from build123d import *

# Parameters (mm, degrees)
SKETCH1_W           = 279.4
SKETCH1_H           = 177.8
BOSS_EXTRUDE1_DEPTH = 25.654
SKETCH9_R           = 3.96875
CUT_EXTRUDE1_DEPTH  = 38.1
SKETCH9_7_R         = 2.5
SKETCH9_7_R_2       = 3.96875
BOSS_EXTRUDE2_DEPTH = 49.53
SKETCH13_W          = 127.6
SKETCH13_H          = 108.000000046
BOSS_EXTRUDE3_DEPTH = 49.53
SKETCH14_W          = 73
SKETCH14_H          = 49.53
BOSS_EXTRUDE4_DEPTH = 30.48
FILLET1_R           = 25.4
FILLET2_R           = 25.4


with BuildPart() as part:
    # Sketch1 → Boss-Extrude1 (new body)
    with BuildSketch(Plane(origin=(0, 0, 0), x_dir=(1, 0, 0), z_dir=(0, 1, 0))):
        with Locations((139.7, 88.9)):
            Rectangle(SKETCH1_W, SKETCH1_H)
    extrude(amount=BOSS_EXTRUDE1_DEPTH)

    # Sketch9 → Cut-Extrude1 (cut)
    with BuildSketch(Plane(origin=(0, 25.654, 0), x_dir=(1, 0, 0), z_dir=(0, 1, 0))):
        with Locations((215, 143)):
            Circle(SKETCH9_R)
    extrude(amount=-CUT_EXTRUDE1_DEPTH, mode=Mode.SUBTRACT)

    # Sketch9<7> → Boss-Extrude2 (add)
    with BuildSketch(Plane(origin=(0, 25.654, 0), x_dir=(1, 0, 0), z_dir=(0, 1, 0))):
        Polygon((0, 108.000000046), (127.6, 108.000000046), (127.6, 0), (280, 0), (280, 178), (0, 178), align=None)
        with Locations((35.318924397, 143)):
            Circle(SKETCH9_7_R, mode=Mode.SUBTRACT)
        with Locations((14, 143)):
            Circle(SKETCH9_7_R_2, mode=Mode.SUBTRACT)
        with Locations((68, 143)):
            Circle(SKETCH9_7_R_2, mode=Mode.SUBTRACT)
        with Locations((270, 167)):
            Circle(SKETCH9_7_R_2, mode=Mode.SUBTRACT)
        with Locations((215, 143)):
            Circle(SKETCH9_7_R_2, mode=Mode.SUBTRACT)
        with BuildLine():
            Line((129.639279667, 129.22), (129.639279667, 126.383968902))
            ThreePointArc((129.639279667, 126.383968902), (148.28, 150), (129.639279667, 173.616031098))
            Line((129.639279667, 173.616031098), (129.639279667, 170.78))
            Line((129.639279667, 170.78), (118.360720333, 170.78))
            Line((118.360720333, 170.78), (118.360720333, 173.616031098))
            ThreePointArc((118.360720333, 173.616031098), (99.72, 150), (118.360720333, 126.383968902))
            Line((118.360720333, 126.383968902), (118.360720333, 129.22))
            Line((118.360720333, 129.22), (129.639279667, 129.22))
        make_face(mode=Mode.SUBTRACT)
    extrude(amount=BOSS_EXTRUDE2_DEPTH)

    # Sketch13 → Boss-Extrude3 (add)
    with BuildSketch(Plane(origin=(0, 25.654, 0), x_dir=(1, 0, 0), z_dir=(0, 1, 0))):
        with Locations((63.8, 54.000000023)):
            Rectangle(SKETCH13_W, SKETCH13_H)
    extrude(amount=BOSS_EXTRUDE3_DEPTH)

    # Sketch14 → Boss-Extrude4 (add)
    with BuildSketch(Plane(origin=(0, 0, -178), x_dir=(-1, 0, 0), z_dir=(0, 0, -1))):
        with Locations((-148.500000008, 50.419)):
            Rectangle(SKETCH14_W, SKETCH14_H)
    extrude(amount=BOSS_EXTRUDE4_DEPTH)

    # Fillet1
    fillet1_edges = [part.edges().sort_by_distance(p)[0] for p in [
        (185.000000008, 50.419, -208.48),
    ]]
    fillet(fillet1_edges, radius=FILLET1_R)

    # Fillet2
    fillet2_edges = [part.edges().sort_by_distance(p)[0] for p in [
        (112.000000008, 50.419, -208.48),
    ]]
    fillet(fillet2_edges, radius=FILLET2_R)


solid = part.part
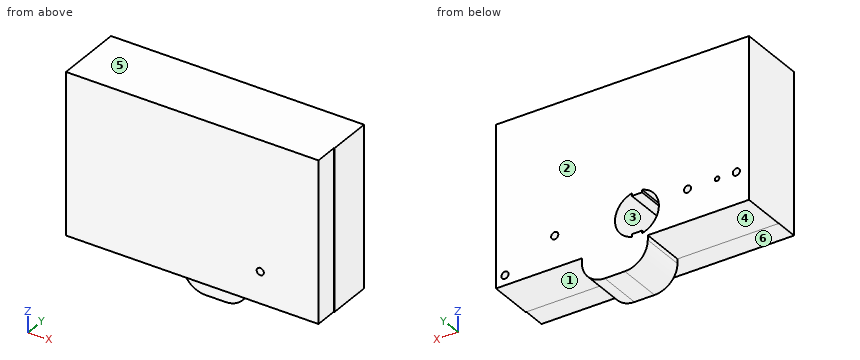
The listing builds one solid part. Answer for the finished solid, in the listing's coordinates (mm). Face numbers are marked on the shaded views. A direction names the side the tool comes from. Coordinates: 2 decimals unless noted, no trailing zeros. Write each loop counter-clockwise with the first axis right and the second up, starting at its lowest first coordinate (ties: lowest second). Pieces come first, ordered by that corner, then holes. Notation, with made-up numbers: M 87,-8 L 117,-8 A23 ccw 117,2 Z; hole C -29,52.25 d9. An arc over 180 degrees is marked long. Put each result on its own line as item: value. Start each with the question number.
1. A cutting plane is placed at B-B on y = 70. Write down the section's boundary in (x, z), then the cut area to 3 significant figures.
2. Consider line 1 (X direction, y = 20, z = -143); line 2 (X direction, y = 46, z = -143); line 3 (Z direction, x = 68, y = 50). Determine where each line is inside the solid, lowest interval first. Write a range as from..to.
3. For a pull along Z with two mould halves and no side action, classify the marked faces 1, 2 and 3 as pulls with the +Z half, pulls with the -Z half, needs draft (parallel to the pull), parting line crosses it, or undercut.
4. A cutting plane is placed at C-C on y = 10.5. Write down the section's boundary in (x, z), then the cut area to 3 significant figures.
5. A cutting plane is placed at A-A on x = 215. Write down the section's boundary in (y, z).
6. Which of the six approach directions +Z, -Z, +X, -X, +Y, -Y give full straight-line access (tool end or side, diameter ignored) to the marked faces 4, 5 and 6?
7. Flat-ended cylindrical pins translate along their axes: P1, Ø15, axis at x = 215, y = 60, coming from the -Z side; P2, Ø5, axis at x = 215, z = -143, coming from the -Y side; P3, Ø20.5, axis at y = 8.5, z = -56, coming from the +X side; P4, Ø4, axis at x = 35.5, z = -143, coming from the +Y side. Find the tip coordinate at first contact, or state that the pin passes through.
8. A cutting plane is placed at D-D on z = -136. Write down the section's boundary in (x, y), then the cut area to 3 significant figures.
Resolved:
1. outline: M 0,-178 L 112,-178 L 112,-183.08 A25.4 ccw 137.4,-208.48 L 159.6,-208.48 A25.4 ccw 185,-183.08 L 185,-178 L 280,-178 L 280,0 L 0,0 Z; hole C 14,-143 d7.94; hole C 35.32,-143 d5; hole C 68,-143 d7.94; hole M 118.36,-173.62 L 118.36,-170.78 L 129.64,-170.78 L 129.64,-173.62 A24.28 ccw 129.64,-126.38 L 129.64,-129.22 L 118.36,-129.22 L 118.36,-126.38 A24.28 ccw Z; hole C 215,-143 d7.94; hole C 270,-167 d7.94
1. area: 49,800 mm2
2. line 1: x = 0..211.03, 218.97..279.4
2. line 2: x = 0..10.03, 17.97..32.82, 37.82..64.03, 71.97..100.75, 147.25..211.03, 218.97..280
2. line 3: z = -178..-146.97, -139.03..0
3. face 1: pulls with the -Z half
3. face 2: needs draft
3. face 3: undercut
4. outline: M 0,-177.8 L 279.4,-177.8 L 279.4,0 L 0,0 Z; hole C 215,-143 d7.94
4. area: 49,600 mm2
5. outline: M 0,-177.8 L 25.65,-177.8 L 25.65,-178 L 75.18,-178 L 75.18,-146.97 L 0,-146.97 Z; M 0,-139.03 L 75.18,-139.03 L 75.18,0 L 0,0 Z
6. face 4: -Z, -X, +Y, -Y
6. face 5: +Z, +X, -X, +Y, -Y
6. face 6: -Z, +X, -X, -Y
7. P1: stops at z = -178
7. P2: passes through
7. P3: stops at x = 279.4
7. P4: stops at y = 25.65
8. outline: M 0,0 L 279.4,0 L 279.4,25.65 L 280,25.65 L 280,75.18 L 143.84,75.18 L 143.84,25.65 L 104.16,25.65 L 104.16,75.18 L 0,75.18 Z
8. area: 19,100 mm2
